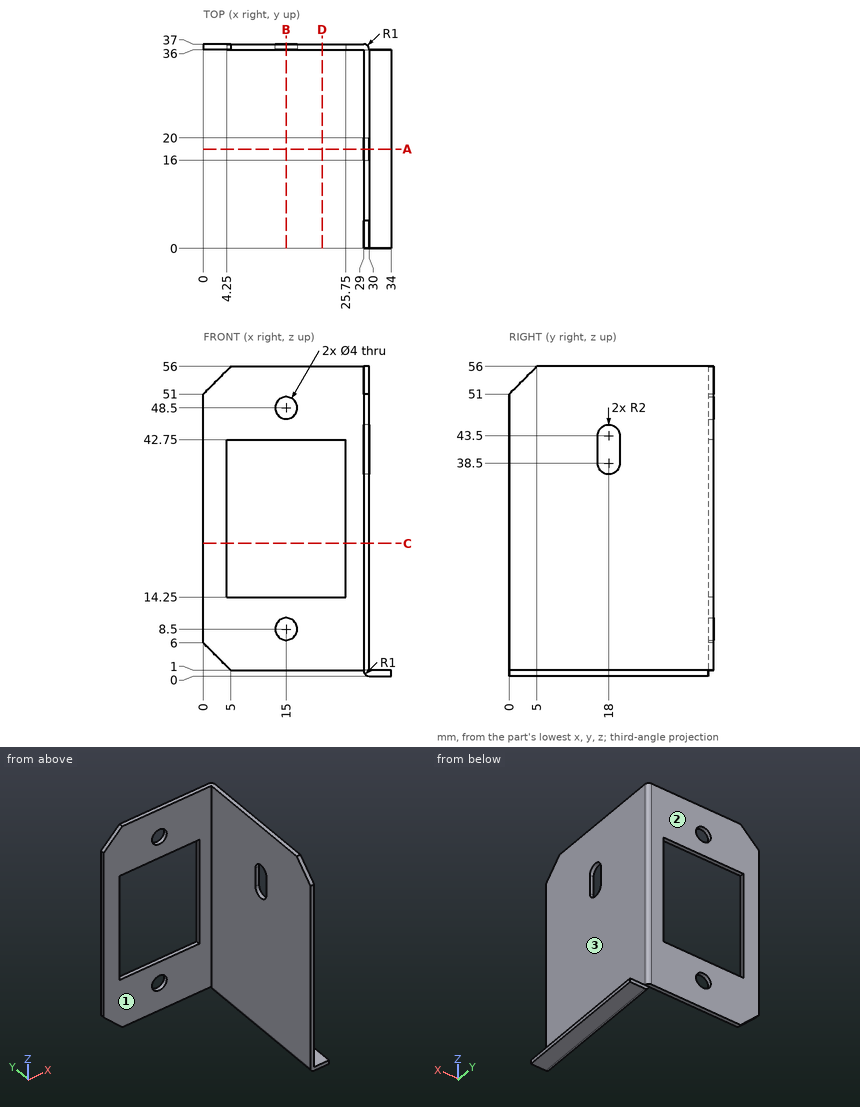
Part print with two shaded views. Sizes in mm from the minimum x, y, z corner. A direction names the side the tool comes from. Give positions to 0.01 mm unless a question says otherwise; leave off trailing zeros. Order: outer loops, then holes, each group sorted by start corner. A loop starts at its lowest first (then second) coordinate and runs counter-clockwise, first axis right, second up.
(1) Saw through at D-D, the plane x = 21.5. Give the cut face in (y, z).
(2) Saw through at A-A, the plane y = 18. Give the cut face in (x, z).
(3) Tool access for the marked faces 1, 2 and 3: list every direction of +Z, -Z, +X, -X, +Y, -Y with a clear straight run to the whole face (end or side of a thin tool).
(4) Flat gauge pins, fed straight in: pin 1 (1.1 mm diameter, centred on x = 32.5, z = 0.5, fed in from +Y); pin 2 (3 mm diameter, centred on x = 3.5, z = 33.5, fed in from -Y); pin 3 (1.1 mm diameter, centred on y = 36.5, z = 23.5, fed in from +X). Where does each tip first touch, or does it go through?
(5) Saw through at C-C, the plane z = 24. Give the cut face in (x, y), then the cut area to 3 significant figures.
(6) Saw through at B-B, the plane x = 15. Give the cut face in (y, z).
(7) Drill centre lines: L1, parallel to Z at x = 15, y = 36.5; L2, parallel to X at y = 29, z = 39; L3, parallel to Y at x = 24, z = 51. Where is each one in solid material? Low to high.
Results found:
1. outline: (36, 1) - (37, 1) - (37, 14.25) - (36, 14.25) - close; (36, 42.75) - (37, 42.75) - (37, 56) - (36, 56) - close
2. outline: (29, 1) arc R1 ccw to (30, 0) - (34, 0) - (34, 1) - (30, 1) - (30, 36.5) - (29, 36.5) - close; (29, 45.5) - (30, 45.5) - (30, 56) - (29, 56) - close
3. face 1: +Z, -Z, -X, -Y
3. face 2: +Z, -Z, +X, -X, +Y
3. face 3: +Z, +X, +Y, -Y
4. pin 1: stops at y = 36
4. pin 2: stops at y = 36
4. pin 3: stops at x = 30
5. outline: (0, 36) - (4.25, 36) - (4.25, 37) - (0, 37) - close; (25.75, 36) - (29, 36) - (29, 0) - (30, 0) - (30, 36) arc R1 ccw to (29, 37) - (25.75, 37) - close
5. area: 44.3 mm2
6. outline: (36, 1) - (37, 1) - (37, 6.5) - (36, 6.5) - close; (36, 10.5) - (37, 10.5) - (37, 14.25) - (36, 14.25) - close; (36, 42.75) - (37, 42.75) - (37, 46.5) - (36, 46.5) - close; (36, 50.5) - (37, 50.5) - (37, 56) - (36, 56) - close
7. L1: z = 1 to 6.5, 10.5 to 14.25, 42.75 to 46.5, 50.5 to 56
7. L2: x = 29 to 30
7. L3: y = 36 to 37
